Input: part model. Units: mm. Frame: model coordinates. A direction names the side the tool comes from. Coordinates: 2 decimals unless noted, no trailing zeros. Loops run counter-clockwise (first coordinate to the right, second up) from the corner with the lowest first, then second, coordinate; pieces in that order, holes last. Notation, with made-up numbers: (30, 13.5) - (36, 13.5) arc R31 cw to (36, 47.5) - close; hole circle Ø10 at (24, 36.25). An arc over 180 degrees is marked (long way). Use a Markdown table: item, result. Add a question column.
1. Section query A-A on y = 22.6. Return the cut outline in (x, z).
2. Contact query for flat-ended pins moving along their axis: P1, Ø1, axis at y = 22, z = -57.5, coming from the +X side; P2, Ø1, axis at y = 23, z = 22.5, coming from the -X side; P3, Ø1, axis at x = -64, y = 22.5, coming from the +Z side. Output: stop coordinate, or through.
3. Section query B-B on z = -57. Return the cut outline in (x, y).
4. Ray query, L1, parallel to X at y = 22.7, z = 13; L2, parallel to X at y = 23, z = -61; L3, parallel to Z at x = -46.5, y = 22.45. Return the intervals inside material, ascending. Write a range as [from, to].
5. Draft query along Z for faces 1 (the face through (-52, 22, 25.5)), 2 (the face through (-60.614, 22.486, -32.385)), 3 (the face through (-60, 22, -52)). Return one class per face: released by +Z, released by -Z, zero draft, split by the parting line, or undercut.
6. Access query for faces 4 (the face through (-44.4, 22, -5)), 5 (the face through (-63, 22, 18)), 6 (the face through (-46, 22, -35.5)), 7 (the face through (-63, 22, -36.8)). Directions: +Z, -Z, +X, -X, +Y, -Y. A direction counts if a zero-diameter tool reaches every point of the face in a straight line with its end or side. Return the directions, or none.
```python
from build123d import *

# Parameters (mm, degrees)
BOSS_EXTRUDE1_DEPTH = 1.5
SKETCH2_W           = 4.8
SKETCH2_H           = 18
BOSS_EXTRUDE2_DEPTH = 20
SKETCH3_R           = 1.5
CUT_EXTRUDE1_DEPTH  = 20
SKETCH4_R           = 3
SKETCH4_R_2         = 1.5
SKETCH4_W           = 4.828517764
SKETCH4_H           = 3.2
SKETCH4_W_2         = 5.829541735
SKETCH4_H_2         = 5.702554953
SKETCH4_W_3         = 4.58984945
BOSS_EXTRUDE3_DEPTH = 3.8
SKETCH5_W           = 7.960049614
SKETCH5_H           = 4.589179968
SKETCH5_R           = 1.5
SKETCH5_W_2         = 8.506770289
SKETCH5_H_2         = 5.091999219
SKETCH5_W_3         = 7.172313144
SKETCH5_H_3         = 12.5
SKETCH5_H_4         = 13
BOSS_EXTRUDE4_DEPTH = 4.25
SKETCH6_W           = 6.917388718
SKETCH6_H           = 7.693263261
SKETCH6_R           = 1.5
SKETCH6_W_2         = 6.017640473
SKETCH6_H_2         = 7.169329529
BOSS_EXTRUDE5_DEPTH = 12.5
SKETCH7_R           = 1.5
BOSS_EXTRUDE7_DEPTH = 2
INTERSECT1_DEPTH    = 21.5


# Read off the part's stored shape, not the designer's step: Intersect1
with BuildPart() as part:
    # Sketch1 → Boss-Extrude1 (new body)
    with BuildSketch(Plane(origin=(0, 0, 0), x_dir=(1, 0, 0), z_dir=(0, 1, 0))):
        Polygon((-60, -67.5), (-60, -72.5), (-52, -72.5), (-52, -67.5), (52, -67.5), (52, -72.5), (60, -72.5), (60, -67.5), (60, 67.5), (-60, 67.5), (-60, 36.8), (-65.5, 36.8), (-65.5, 29.3), (-60, 29.3), (-60, 16.8), (-65.5, 16.8), (-65.5, 7.8), (-65.5, -1.2), (-60, -1.2), (-60, -10.5), (-65.5, -10.5), (-65.5, -18), (-60, -18), align=None)
    extrude(amount=BOSS_EXTRUDE1_DEPTH)

    # Sketch2 → Boss-Extrude2 (add)
    with BuildSketch(Plane(origin=(0, 1.5, 0), x_dir=(1, 0, 0), z_dir=(0, 1, 0))):
        Polygon((-58, 62.8), (-58, 29.3), (-60, 29.3), (-65.5, 29.3), (-65.5, 36.8), (-60, 36.8), (-60, 67.5), (-55.3, 67.5), (-55.3, 65.5), align=None)
        with BuildLine():
            Line((-58, -65.5), (58, -65.5))
            Line((58, -65.5), (58, -25.5))
            Line((58, -25.5), (29.8, -25.5))
            Line((29.8, -25.5), (29.8, -18))
            Line((29.8, -18), (58, -18))
            Line((58, -18), (58, 38.5))
            ThreePointArc((58, 38.5), (57.414213562, 39.914213562), (56, 40.5))
            Line((56, 40.5), (51.8, 40.5))
            ThreePointArc((51.8, 40.5), (50.385786438, 41.085786438), (49.8, 42.5))
            Line((49.8, 42.5), (49.8, 48.75))
            Line((49.8, 48.75), (51.3, 48.75))
            Line((51.3, 48.75), (51.3, 47.25))
            Line((51.3, 47.25), (58, 47.25))
            Line((58, 47.25), (58, 51.25))
            Line((58, 51.25), (60, 51.25))
            Line((60, 51.25), (60, -72.5))
            Line((60, -72.5), (52, -72.5))
            Line((52, -72.5), (52, -67.5))
            Line((52, -67.5), (-52, -67.5))
            Line((-52, -67.5), (-52, -72.5))
            Line((-52, -72.5), (-60, -72.5))
            Line((-60, -72.5), (-60, -52.5))
            Line((-60, -52.5), (-58, -52.5))
            Line((-58, -52.5), (-58, -65.5))
        make_face()
        Polygon((-60, 16.8), (-58, 16.8), (-58, -1.2), (-60, -1.2), (-65.5, -1.2), (-65.5, 16.8), align=None)
        Polygon((-60, -10.5), (-58, -10.5), (-58, -38), (-60, -38), (-60, -18), (-65.5, -18), (-65.5, -10.5), align=None)
        with BuildLine():
            Line((-48.8, 67.5), (-48.8, 65.5))
            Line((-48.8, 65.5), (-46.8, 62.8))
            Line((-46.8, 62.8), (-46.8, 58.5))
            Line((-46.8, 58.5), (-44.8, 58.5))
            Line((-44.8, 58.5), (-37.8, 64.5))
            Line((-37.8, 64.5), (38.8, 64.5))
            Line((38.8, 64.5), (44.8, 58.5))
            Line((44.8, 58.5), (44.8, 46.5))
            Line((44.8, 46.5), (41.3, 46.5))
            Line((41.3, 46.5), (41.3, 42.5))
            Line((41.3, 42.5), (38.85, 42.5))
            Line((38.85, 42.5), (38.85, 40.5))
            Line((38.85, 40.5), (44.8, 40.5))
            ThreePointArc((44.8, 40.5), (46.214213562, 41.085786438), (46.8, 42.5))
            Line((46.8, 42.5), (46.8, 46.5))
            Line((46.8, 46.5), (46.8, 57.25))
            Line((46.8, 57.25), (51.3, 57.25))
            Line((51.3, 57.25), (51.3, 58.75))
            Line((51.3, 58.75), (58, 58.75))
            Line((58, 58.75), (58, 54.75))
            Line((58, 54.75), (60, 54.75))
            Line((60, 54.75), (60, 67.5))
            Line((60, 67.5), (-48.8, 67.5))
        make_face()
        Polygon((-46.8, 46.5), (-39.5, 46.5), (-39.5, 42.5), (-37.05, 42.5), (-37.05, 40.5), (-46.8, 40.5), align=None)
        Polygon((-33.55, 42.5), (-33.55, 40.5), (-18.65, 40.5), (-18.65, 42.5), (-21.1, 42.5), (-21.1, 46.5), (-31.1, 46.5), (-31.1, 42.5), align=None)
        Polygon((-15.55, 40.5), (-0.65, 40.5), (-0.65, 42.5), (-3.1, 42.5), (-3.1, 46.5), (-13.1, 46.5), (-13.1, 42.5), (-15.55, 42.5), align=None)
        Polygon((2.45, 40.5), (17.35, 40.5), (17.35, 42.5), (14.9, 42.5), (14.9, 46.5), (4.9, 46.5), (4.9, 42.5), (2.45, 42.5), align=None)
        Polygon((20.45, 40.5), (35.35, 40.5), (35.35, 42.5), (32.9, 42.5), (32.9, 46.5), (22.9, 46.5), (22.9, 42.5), (20.45, 42.5), align=None)
        Polygon((-46.8, 35.5), (-49.2, 35.5), (-49.2, 29.3), (-44.4, 29.3), (-44.4, 35.5), align=None)
        with Locations((-46.8, 7.8)):
            Rectangle(SKETCH2_W, SKETCH2_H)
        Polygon((-49.2, -10.5), (-44.4, -10.5), (-44.4, -18), (-16.9, -18), (-16.9, -25.5), (-46.4, -25.5), (-46.4, -19.9), (-49.2, -14), align=None)
    extrude(amount=BOSS_EXTRUDE2_DEPTH)

    # Sketch3 → Cut-Extrude1 (cut)
    with BuildSketch(Plane(origin=(0, 21.5, 0), x_dir=(1, 0, 0), z_dir=(0, 1, 0))):
        with Locations(Location((52.774715074, 63.354517547, 0), (0, 0, 270))):
            Circle(SKETCH3_R)
        with Locations(Location((-43.84271688, 64.854517547, 0), (0, 0, 270))):
            Circle(SKETCH3_R)
        with Locations(Location((-61.879270776, 33.191143968, 0), (0, 0, 270))):
            Circle(SKETCH3_R)
        with Locations(Location((-61.879270776, -14.337618299, 0), (0, 0, 270))):
            Circle(SKETCH3_R)
        with Locations(Location((54.274715074, 43.945098524, 0), (0, 0, 270))):
            Circle(SKETCH3_R)
        with Locations(Location((-21.029637868, -21.862387391, 0), (0, 0, 270))):
            Circle(SKETCH3_R)
        with Locations(Location((34.3, -21.75, 0), (0, 0, 270))):
            Circle(SKETCH3_R)
        with Locations(Location((-56, -69, 0), (0, 0, 270))):
            Circle(SKETCH3_R)
        with Locations(Location((56, -69, 0), (0, 0, 270))):
            Circle(SKETCH3_R)
    extrude(amount=-CUT_EXTRUDE1_DEPTH, mode=Mode.SUBTRACT)

    # Sketch4 → Boss-Extrude3 (add)
    # profile 1 of 5: a face of its own
    with BuildSketch(Plane(origin=(0, 1.5, 0), x_dir=(1, 0, 0), z_dir=(0, 1, 0))):
        with Locations(Location((21.544764921, -8.320497528, 0), (0, 0, 90))):
            Circle(SKETCH4_R)
        with Locations(Location((21.544764921, -8.320497528, 0), (0, 0, 90))):
            Circle(SKETCH4_R_2, mode=Mode.SUBTRACT)
    # profile 2 of 5: a face of its own
    with BuildSketch(Plane(origin=(0, 1.5, 0), x_dir=(1, 0, 0), z_dir=(0, 1, 0))):
        with Locations(Location((21.544764921, 19.479502472, 0), (0, 0, 90))):
            Circle(SKETCH4_R)
        with Locations(Location((21.544764921, 19.479502472, 0), (0, 0, 90))):
            Circle(SKETCH4_R_2, mode=Mode.SUBTRACT)
    # profile 3 of 5: a face of its own
    with BuildSketch(Plane(origin=(0, 1.5, 0), x_dir=(1, 0, 0), z_dir=(0, 1, 0))):
        with Locations((-29.2, 33.9)):
            Rectangle(SKETCH4_W, SKETCH4_H)
        with Locations(Location((-29.2, 33.9, 0), (0, 0, 90))):
            Circle(SKETCH4_R_2, mode=Mode.SUBTRACT)
    # profile 4 of 5: a face of its own
    with BuildSketch(Plane(origin=(0, 1.5, 0), x_dir=(1, 0, 0), z_dir=(0, 1, 0))):
        with Locations((-30.25253813, -15.148722524)):
            Rectangle(SKETCH4_W_2, SKETCH4_H_2)
        with Locations(Location((-30.3, -14.4, 0), (0, 0, 90))):
            Circle(SKETCH4_R_2, mode=Mode.SUBTRACT)
    # profile 5 of 5: a face of its own
    with BuildSketch(Plane(origin=(0, 1.5, 0), x_dir=(1, 0, 0), z_dir=(0, 1, 0))):
        with Locations((51.718864017, -15.148722524)):
            Rectangle(SKETCH4_W_3, SKETCH4_H_2)
        with Locations(Location((51.8, -14.4, 0), (0, 0, 90))):
            Circle(SKETCH4_R_2, mode=Mode.SUBTRACT)
    extrude(amount=BOSS_EXTRUDE3_DEPTH)

    # Sketch5 → Boss-Extrude4 (add)
    # profile 1 of 4: a face of its own
    with BuildSketch(Plane(origin=(0, 1.5, 0), x_dir=(1, 0, 0), z_dir=(0, 1, 0))):
        with Locations((-54.019975193, -35.705410016)):
            Rectangle(SKETCH5_W, SKETCH5_H)
        with Locations(Location((-52.773553759, -35.8, 0), (0, 0, 270))):
            Circle(SKETCH5_R, mode=Mode.SUBTRACT)
    # profile 2 of 4: a face of its own
    with BuildSketch(Plane(origin=(0, 1.5, 0), x_dir=(1, 0, 0), z_dir=(0, 1, 0))):
        with Locations((-53.746614856, -55.04599961)):
            Rectangle(SKETCH5_W_2, SKETCH5_H_2)
        with Locations(Location((-52.773553759, -54.7, 0), (0, 0, 270))):
            Circle(SKETCH5_R, mode=Mode.SUBTRACT)
    # profile 3 of 4: a face of its own
    with BuildSketch(Plane(origin=(0, 1.5, 0), x_dir=(1, 0, 0), z_dir=(0, 1, 0))):
        with Locations((-27.40354529, -31.75)):
            Rectangle(SKETCH5_W_3, SKETCH5_H_3)
        with Locations(Location((-27.173553759, -35.8, 0), (0, 0, 270))):
            Circle(SKETCH5_R, mode=Mode.SUBTRACT)
    # profile 4 of 4: a face of its own
    with BuildSketch(Plane(origin=(0, 1.5, 0), x_dir=(1, 0, 0), z_dir=(0, 1, 0))):
        with Locations((-27.40354529, -59)):
            Rectangle(SKETCH5_W_3, SKETCH5_H_4)
        with Locations(Location((-27.173553759, -54.7, 0), (0, 0, 270))):
            Circle(SKETCH5_R, mode=Mode.SUBTRACT)
    extrude(amount=BOSS_EXTRUDE4_DEPTH)

    # Sketch6 → Boss-Extrude5 (add)
    # profile 1 of 4: a face of its own
    with BuildSketch(Plane(origin=(0, 1.5, 0), x_dir=(1, 0, 0), z_dir=(0, 1, 0))):
        with Locations((-20.358694359, -29.346631631)):
            Rectangle(SKETCH6_W, SKETCH6_H)
        with Locations(Location((-19.26, -30.5, 0), (0, 0, 270))):
            Circle(SKETCH6_R, mode=Mode.SUBTRACT)
    # profile 2 of 4: a face of its own
    with BuildSketch(Plane(origin=(0, 1.5, 0), x_dir=(1, 0, 0), z_dir=(0, 1, 0))):
        with Locations((54.991179763, -29.346631631)):
            Rectangle(SKETCH6_W_2, SKETCH6_H)
        with Locations(Location((55.14, -30.5, 0), (0, 0, 270))):
            Circle(SKETCH6_R, mode=Mode.SUBTRACT)
    # profile 3 of 4: a face of its own
    with BuildSketch(Plane(origin=(0, 1.5, 0), x_dir=(1, 0, 0), z_dir=(0, 1, 0))):
        with Locations((54.991179763, -61.915335236)):
            Rectangle(SKETCH6_W_2, SKETCH6_H_2)
        with Locations(Location((55.14, -61.1, 0), (0, 0, 270))):
            Circle(SKETCH6_R, mode=Mode.SUBTRACT)
    # profile 4 of 4: a face of its own
    with BuildSketch(Plane(origin=(0, 1.5, 0), x_dir=(1, 0, 0), z_dir=(0, 1, 0))):
        with Locations((-20.358694359, -61.915335236)):
            Rectangle(SKETCH6_W, SKETCH6_H_2)
        with Locations(Location((-19.26, -61.1, 0), (0, 0, 270))):
            Circle(SKETCH6_R, mode=Mode.SUBTRACT)
    extrude(amount=BOSS_EXTRUDE5_DEPTH)

    # Intersect1 outline → Intersect1 (cut)
    with BuildSketch(Plane(origin=(0, 0, 0), x_dir=(1, 0, 0), z_dir=(0, 1, 0))):
        Polygon((-60, -72.5), (-52, -72.5), (-52, -67.5), (52, -67.5), (52, -72.5), (60, -72.5), (60, 67.5), (-60, 67.5), (-60, 36.8), (-65.5, 36.8), (-65.5, 29.3), (-60, 29.3), (-60, 16.8), (-65.5, 16.8), (-65.5, -1.2), (-60, -1.2), (-60, -10.5), (-65.5, -10.5), (-65.5, -18), (-60, -18), align=None)
    extrude(amount=INTERSECT1_DEPTH, mode=Mode.SUBTRACT)


with BuildPart() as body_2:
    # Sketch7 → Boss-Extrude7 (new body)
    with BuildSketch(Plane(origin=(0, 21.5, 0), x_dir=(1, 0, 0), z_dir=(0, 1, 0))):
        Polygon((-60, 67.5), (-60, 36.8), (-65.5, 36.8), (-65.5, -18), (-60, -18), (-60, -25.5), (-46.4, -25.5), (-44.4, -25.5), (-44.4, -10.5), (-44.4, 35.5), (-46.8, 35.5), (-46.8, 62.8), (-46.8, 67.5), align=None)
        with Locations(Location((-61.879270776, -14.337618299, 0), (0, 0, 270))):
            Circle(SKETCH7_R, mode=Mode.SUBTRACT)
        with Locations(Location((-61.879270776, 33.191143968, 0), (0, 0, 270))):
            Circle(SKETCH7_R, mode=Mode.SUBTRACT)
    extrude(amount=BOSS_EXTRUDE7_DEPTH)


solid = body_2.part
```
Resolved:
| question | item | result |
|---|---|---|
| 1 | outline | (-65.5, -36.8) - (-60, -36.8) - (-60, -67.5) - (-46.8, -67.5) - (-46.8, -35.5) - (-44.4, -35.5) - (-44.4, 25.5) - (-60, 25.5) - (-60, 18) - (-65.5, 18) - close; hole circle Ø3 at (-61.88, -33.19); hole circle Ø3 at (-61.88, 14.34) |
| 2 | P1 | x = -46.8 |
| 2 | P2 | x = -60 |
| 2 | P3 | z = 18 |
| 3 | outline | (-60, 21.5) - (-46.8, 21.5) - (-46.8, 23.5) - (-60, 23.5) - close |
| 4 | L1 | [-65.5, -62.56], [-61.2, -44.4] |
| 4 | L2 | [-60, -46.8] |
| 4 | L3 | [-35.5, 25.5] |
| 5 | face 1 | released by +Z |
| 5 | face 2 | undercut |
| 5 | face 3 | zero draft |
| 6 | face 4 | +Z, -Z, +X, +Y, -Y |
| 6 | face 5 | +Z, -X, +Y, -Y |
| 6 | face 6 | -Z, +X, +Y, -Y |
| 6 | face 7 | -Z, -X, +Y, -Y |
